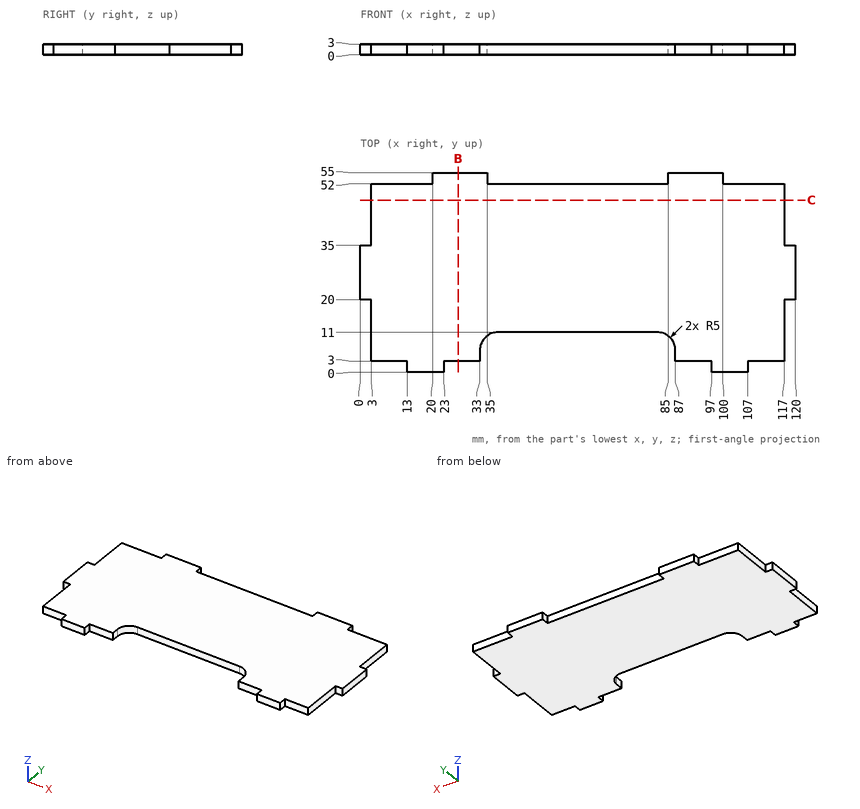
Source: three-view drawing plus pictorial views. Frame: mm from the lowest corner of the part. Give positions to 0.01 mm unless a question says otherwise; leave off trailing zeros. Order: outer loops, then holes, each group sorted by start corner. A loop starts at its lowest first (then second) coordinate and runs counter-clockwise, first axis right, second up. Notation, with made-up numbers: (13.25, -32) -> (51.25, -32) arc R14 cw to (51.25, -11) -> close; hole circle Ø5 at (-37.5, 53.5). An arc over 180 degrees is marked (long way). Use a Markdown table: item, result.
Q1. First-contact query: P1, Ø1.5, axis at x = 2, z = 1, coming from the -Y side; P2, Ø1.5, axis at x = 1.5, z = 2, coming from the +Y side; P3, Ø0.9, axis at y = 53.5, z = 1, coming from the -X side. Flat tips, straight axial feed; report the tip coordinate or a pass-through.
A:
| item | result |
|---|---|
| P1 | y = 20 |
| P2 | y = 35 |
| P3 | x = 20 |
Q2. Section B-B (x = 27). Return the cut outline in (y, z), and give its area (3 significant figures).
A:
| item | result |
|---|---|
| outline | (3, 0) -> (55, 0) -> (55, 3) -> (3, 3) -> close |
| area | 156 mm^2 |
Q3. Material intervals for line 1 (X direction, y = 4.5, z = 0.3); line 2 (X direction, y = 53, z = 2.8); line 3 (Y direction, x = 25, z = 1.7), sorted ascending. Write a range as [from, to].
A:
| item | result |
|---|---|
| line 1 | [3, 33], [87, 117] |
| line 2 | [20, 35], [85, 100] |
| line 3 | [3, 55] |
Q4. Section C-C (y = 47.5). Return the cut outline in (x, z), and give its area (3 significant figures).
A:
| item | result |
|---|---|
| outline | (3, 0) -> (117, 0) -> (117, 3) -> (3, 3) -> close |
| area | 342 mm^2 |
